```python
from build123d import *

# Parameters (mm, degrees)
SKETCH1_W               = 40
SKETCH1_H               = 40
BOSS_EXTRUDE1_DEPTH     = 40
SKETCH2_R               = 1.7
BOSS_EXTRUDE2_DEPTH     = 5
MIRROR2_COPY_1_SKETCH_R = 1.7
MIRROR2_COPY_1_DEPTH    = 5
SKETCH3_R               = 2.5
BOSS_EXTRUDE3_DEPTH     = 20


with BuildPart() as part:
    # Sketch1 → Boss-Extrude1 (new body)
    with BuildSketch(Plane.XY):
        Rectangle(SKETCH1_W, SKETCH1_H)
    extrude(amount=BOSS_EXTRUDE1_DEPTH)

    # Sketch2 → Boss-Extrude2 (add)
    with BuildSketch(Plane(origin=(0, 0, 0), x_dir=(-1, 0, 0), z_dir=(0, 0, -1))):
        with Locations((15, -15)):
            Circle(SKETCH2_R)
    boss_extrude2 = extrude(amount=BOSS_EXTRUDE2_DEPTH)

    # Mirror1: Boss-Extrude2 across plane
    add(boss_extrude2.mirror(Plane(origin=(0, 0, 0), x_dir=(0, 0, 1), z_dir=(1, 0, 0))))

    # Mirror2: Boss-Extrude2 across plane
    add(boss_extrude2.mirror(Plane.ZX))

    # Mirror2 copy 1 sketch → Mirror2 copy 1 (add)
    with BuildSketch(Plane(origin=(0, 0, 0), x_dir=(1, 0, 0), z_dir=(0, 0, -1))):
        with Locations((15, -15)):
            Circle(MIRROR2_COPY_1_SKETCH_R)
    extrude(amount=MIRROR2_COPY_1_DEPTH)

    # Sketch3 → Boss-Extrude3 (add)
    with BuildSketch(Plane(origin=(0, 0, 0), x_dir=(-1, 0, 0), z_dir=(0, 0, -1))):
        Circle(SKETCH3_R)
    extrude(amount=BOSS_EXTRUDE3_DEPTH)


solid = part.part
```
Here's how the part is built. I have some questions about the finished solid (model axes, mm). A direction names the side the tool comes from. Coordinates: 2 decimals unless noted, no trailing zeros. Write each loop counter-clockwise with the first axis right and the second up, starting at its lowest first coordinate (ties: lowest second). Pieces come first, ordered by that corner, then holes. Notation, with made-up numbers: (64, 42.5) - (105, 42.5) arc R26 ccw to (105, 76.5) - close; hole circle Ø9 at (-32.5, 15). An arc over 180 degrees is marked (long way). One line per item, written item: value.
1) We'd pull the mould along Y, two halves only. Please class faces 1 (the flat face through (0, 0, 40)), 2 (the flat face through (0, 20, 20)), 3 (the flat face through (0, -20, 20)), 4 (the cylindrical face through (16.57, -15.65, -2.46)): pulls with the +Y half, pulls with the -Y half, needs draft (parallel to the pull), parting line crosses it, or undercut.
Model answer:
face 1: needs draft
face 2: pulls with the +Y half
face 3: pulls with the -Y half
face 4: undercut
2) Suppose I cut it at B-B on z = -1. Write out the boundary of the cut face in (x, y).
Model answer:
outline: circle Ø3.4 at (-15, -15); circle Ø3.4 at (-15, 15); circle Ø5 at (0, 0); circle Ø3.4 at (15, -15); circle Ø3.4 at (15, 15)
3) Suppose I cut it at D-D on z = -12. Write out the boundary of the cut face in (x, y), and give its area (3 significant figures).
Model answer:
outline: circle Ø5 at (0, 0)
area: 19.6 mm²
4) I'm going to push flat-ended pins straight in: P1, Ø2.5, axis at x = -15.5, y = 15.5, coming from the -Z side; P2, Ø4, axis at x = 13.5, y = -10.5, coming from the -Z side. Where does each tip first touch, or does it pass through?
Model answer:
P1: stops at z = -5
P2: stops at z = 0
5) On a 3-axis mill with a long thin cutter (end or side, diameter ignored), from which of +Z, -Z, +X, -X, +Y, -Y can I reach the whole of each face in a straight line? I mean faces 5 (the flat face through (-20, 0, 20)), 6 (the cylindrical face through (0.54, -2.44, -9.86)). Say none if no direction works.
Model answer:
face 5: +Z, -Z, -X, +Y, -Y
face 6: -Z
6) Suppose I cut it at C-C on y = 15. Write out the boundary of the cut face in (x, z).
Model answer:
outline: (-20, 0) - (-16.7, 0) - (-16.7, -5) - (-13.3, -5) - (-13.3, 0) - (13.3, 0) - (13.3, -5) - (16.7, -5) - (16.7, 0) - (20, 0) - (20, 40) - (-20, 40) - close
7) Suppose I cut it at A-A on x = 0. Write out the boundary of the cut face in (y, z), and give its area (3 significant figures).
Model answer:
outline: (-20, 0) - (-2.5, 0) - (-2.5, -20) - (2.5, -20) - (2.5, 0) - (20, 0) - (20, 40) - (-20, 40) - close
area: 1,700 mm²
8) I need wall thicknesses on line 1 along Z through (x, y) = (6, 16.5); line 2 along Y through (x, z) = (14, -1). Which ranges of each line are inside material? Lowest first, please.
Model answer:
line 1: z = 0 to 40
line 2: y = -16.37 to -13.63, 13.63 to 16.37
